Check sheet for the modelled part. Datum: model origin and axes. Units: mm. A direction names the side the tool comes from. Round coordinates to 2 decimals unless told otherwise and drop trailing zeros. Loops run counter-clockwise (first coordinate to the right, second up) from the corner with the lowest first, then second, coordinate; pieces in that order, holes last. Notation, with made-up numbers: (-22, -35) -> (22, -35) arc R15 cw to (22, -16) -> close; hole circle Ø5 at (-30.5, 88.5). An arc over 180 degrees is marked (long way). One line per question, with ' | ' between items.
```python
from build123d import *

# Parameters (mm, degrees)
SKETCH1_R           = 177
SKETCH1_R_2         = 1.5
BOSS_EXTRUDE1_DEPTH = 6.35


with BuildPart() as part:
    # Sketch1 → Boss-Extrude1 (new body)
    with BuildSketch(Plane(origin=(0, 0, 0), x_dir=(1, 0, 0), z_dir=(0, 1, 0))):
        with Locations(Location((0, 0, 0), (0, 0, 270))):
            Circle(SKETCH1_R)
        with Locations(Location((-101.6, -101.6, 0), (0, 0, 270))):
            Circle(SKETCH1_R_2, mode=Mode.SUBTRACT)
        with Locations(Location((-101.6, 101.6, 0), (0, 0, 270))):
            Circle(SKETCH1_R_2, mode=Mode.SUBTRACT)
        with Locations(Location((101.6, 101.6, 0), (0, 0, 270))):
            Circle(SKETCH1_R_2, mode=Mode.SUBTRACT)
        with Locations(Location((101.6, -101.6, 0), (0, 0, 270))):
            Circle(SKETCH1_R_2, mode=Mode.SUBTRACT)
        with Locations(Location((-127, 76.2, 0), (0, 0, 270))):
            Circle(SKETCH1_R_2, mode=Mode.SUBTRACT)
        with Locations(Location((127, 76.2, 0), (0, 0, 270))):
            Circle(SKETCH1_R_2, mode=Mode.SUBTRACT)
        with Locations(Location((127, -76.2, 0), (0, 0, 270))):
            Circle(SKETCH1_R_2, mode=Mode.SUBTRACT)
        with Locations(Location((-127, -76.2, 0), (0, 0, 270))):
            Circle(SKETCH1_R_2, mode=Mode.SUBTRACT)
        with BuildLine():
            Line((-76.375196212, 152.726666572), (-51.943188071, 161.619190299))
            ThreePointArc((-51.943188071, 161.619190299), (-44.29680402, 161.285341961), (-39.12606043, 155.642465524))
            Line((-39.12606043, 155.642465524), (-38.1, 152.823387662))
            ThreePointArc((-38.1, 152.823387662), (-38.433848337, 145.177003611), (-44.076724775, 140.006260021))
            Line((-44.076724775, 140.006260021), (-68.508732915, 131.113736294))
            ThreePointArc((-68.508732915, 131.113736294), (-76.155116966, 131.447584632), (-81.325860556, 137.090461069))
            Line((-81.325860556, 137.090461069), (-82.351920986, 139.909538931))
            ThreePointArc((-82.351920986, 139.909538931), (-82.018072649, 147.555922982), (-76.375196212, 152.726666572))
        make_face(mode=Mode.SUBTRACT)
        with BuildLine():
            Line((51.943188071, 161.619190299), (76.375196212, 152.726666572))
            ThreePointArc((76.375196212, 152.726666572), (82.018072649, 147.555922982), (82.351920986, 139.909538931))
            Line((82.351920986, 139.909538931), (81.325860556, 137.090461069))
            ThreePointArc((81.325860556, 137.090461069), (76.155116966, 131.447584632), (68.508732915, 131.113736294))
            Line((68.508732915, 131.113736294), (44.076724775, 140.006260021))
            ThreePointArc((44.076724775, 140.006260021), (38.433848337, 145.177003611), (38.1, 152.823387662))
            Line((38.1, 152.823387662), (39.12606043, 155.642465524))
            ThreePointArc((39.12606043, 155.642465524), (44.29680402, 161.285341961), (51.943188071, 161.619190299))
        make_face(mode=Mode.SUBTRACT)
    extrude(amount=BOSS_EXTRUDE1_DEPTH)


solid = part.part
```
(1) Scan lines: probe 1 along X at (y, z) = (5.75, -76); probe 2 along Z at (x, y) = (-127, 3.25); probe 3 along Z at (x, y) = (101, 2.25). Record each from-to range of solid material in increasing order.
Answer:
probe 1: x = -159.85 to -128.49, -125.51 to 125.51, 128.49 to 159.85 | probe 2: z = -123.29 to -77.7, -74.7 to 74.7, 77.7 to 123.29 | probe 3: z = -145.35 to -102.97, -100.23 to 100.23, 102.97 to 145.35
(2) Sectioned sample at A-A, the plane y = 2.5. Count the separate pieces of the cut face and the enclosed holes in it, and give its area (3 significant figures).
Answer:
separate pieces: 1 | enclosed holes: 10 | area: 96,400 mm2
(3) Set-up check for faces 1 (the face through (-64.33, 3.13, -157.11)), 2 (the face through (2, 0, -2)): record each of +Z, -Z, +X, -X, +Y, -Y from which the full face is reachable in a straight line by a thin tool's end or side.
Answer:
face 1: +Y, -Y | face 2: +Z, -Z, +X, -X, -Y
(4) Go/stop test with flat-tipped pins: pin 1 (8 mm diameter, centred on x = -31.5, z = 50, fed in from -Y); pin 2 (2 mm diameter, centred on x = -73.5, y = 1.5, fed in from +Z); pin 3 (1 mm diameter, centred on x = -100, y = 4, fed in from -Z); pin 4 (3 mm diameter, centred on x = 36, y = 4.5, fed in from +Z). Record where each tip stops, or that it passes through.
Answer:
pin 1: stops at y = 0 | pin 2: stops at z = 161.47 | pin 3: stops at z = -146.39 | pin 4: stops at z = 173.61
(5) Sectioned sample at B-B, the plane x = -109.5. Record the cut outline in (y, z).
Answer:
outline: (0, -139.06) -> (6.35, -139.06) -> (6.35, 139.06) -> (0, 139.06) -> close
(6) Sectioned sample at C-C, the plane z = -55. Record the cut outline in (x, y), and give its area (3 significant figures).
Answer:
outline: (-168.24, 0) -> (168.24, 0) -> (168.24, 6.35) -> (-168.24, 6.35) -> close | area: 2,140 mm2
(7) Mould release check, pull along Z, two halves, no side actions. Record for faces 3 (the face through (-172.79, 3.13, -38.37)), 4 (the face through (56.46, 3.13, -135.5)), 5 (the face through (2, 6.35, -2)): +Z half, -Z half, draft (parallel to the pull), parting line (faces both ways), or undercut.
Answer:
face 3: parting line | face 4: undercut | face 5: draft
